For this review, use the dimensioned drawing (mm, ordinates from the lowest corner) and the shaded views. Give positions to 0.01 mm unless a question says otherwise; leave off trailing zeros. Order: outer loops, then holes, each group sorted by start corner. A loop starts at its lowest first (then second) coordinate and runs counter-clockwise, first axis right, second up. Notation, with made-up numbers: M 11,-5 L 62,-5 A26 ccw 62,32 Z; hole C 51.5,33.25 d3. An arc over 180 degrees is marked long. Use CSV: the item, a comma, the result in double quotes. Start each with the question number.
(1) Draft analysis for pull direction Z (two halves, no side actions). For the marked faces 1, 2, 3 and 4, state which applies: pulls with the +Z half, pulls with the -Z half, needs draft (parallel to the pull), parting line crosses it, or undercut.
(2) Wall thickness on L1, parallel to Z at x = 2.95, y = 12; L2, parallel to X at y = 1.5, z = 3.6 (1 decimal); L3, parallel to X at y = 2, z = 3.1 (1 decimal): over which ranges is each line inside the solid? List them lowest first. Write a range as from..to.
(3) Consider section C-C (z = 1.9). Write out the cut boundary in (x, y).
(4) Consider section A-A (x = 4.15). Write out the cut boundary in (y, z).
(5) Consider section D-D (z = 0.4). Write out the cut boundary in (x, y).
(6) Clearance check with flat-ended pins moving along their axes: P1, Ø1.5, axis at y = 13.5, z = 1.5, coming from the +X side; P2, Ø2, axis at y = 10, z = 3, coming from the -X side; P3, Ø1.5, axis at y = 6, z = 1.5, coming from the -X side (1 decimal). State where each tip first meets the part, or that it passes through.
(7) Consider section B-B (y = 4). Write out the cut boundary in (x, z), and give its area (3 significant figures).
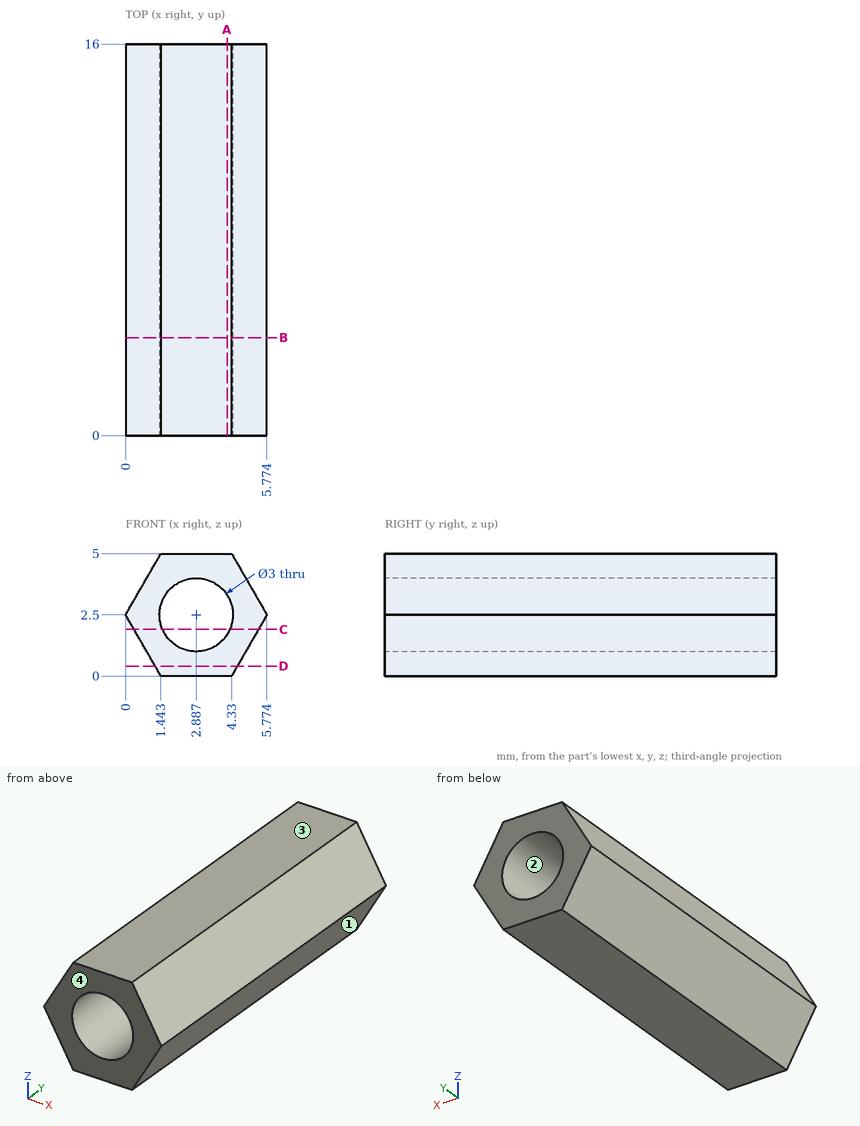
Check result:
1,face 1,"pulls with the -Z half"
1,face 2,"undercut"
1,face 3,"pulls with the +Z half"
1,face 4,"needs draft"
2,L1,"z = 0..1, 4..5"
2,L2,"x = 0.6..1.9, 3.9..5.1"
2,L3,"x = 0.3..1.5, 4.3..5.4"
3,outline,"M 0.35,0 L 1.51,0 L 1.51,16 L 0.35,16 Z; M 4.26,0 L 5.43,0 L 5.43,16 L 4.26,16 Z"
4,outline,"M 0,0 L 16,0 L 16,1.69 L 0,1.69 Z; M 0,3.31 L 16,3.31 L 16,5 L 0,5 Z"
5,outline,"M 1.21,0 L 4.56,0 L 4.56,16 L 1.21,16 Z"
6,P1,"stops at x = 5.63"
6,P2,"stops at x = 0"
6,P3,"stops at x = 0.1"
7,outline,"M 0,2.5 L 1.44,0 L 4.33,0 L 5.77,2.5 L 4.33,5 L 1.44,5 Z; hole C 2.89,2.5 d3"
7,area,"14.6 mm^2"
